```python
from build123d import *

# Parameters (mm, degrees)
SKIZZE1_W   = 5
SKIZZE1_H   = 80
SKIZZE1_W_2 = 50
SKIZZE1_H_2 = 5


with BuildPart() as part:
    # Skizze1 → Rotation1 (revolve)
    with BuildSketch(Plane.XY, mode=Mode.PRIVATE) as rotation1_sk:
        with Locations((-2.5, 40)):
            Rectangle(SKIZZE1_W, SKIZZE1_H)
        with Locations((25, 72.5)):
            Rectangle(SKIZZE1_W_2, SKIZZE1_H_2)
    revolve(rotation1_sk.sketch.rotate(Axis((0, 0, 0), (1, 0, 0)), 90), axis=Axis((0, 0, 0), (1, 0, 0)))


solid = part.part
```
Build history of the part. All positions in model axes, mm. A direction names the side the tool comes from. Give positions to 0.01 mm unless a question says otherwise; leave off trailing zeros. Loops run counter-clockwise (first coordinate to the right, second up) from the corner with the lowest first, then second, coordinate; pieces in that order, holes last.
Item 1: Flat gauge pins, fed straight in: pin 1 (6 mm diameter, centred on y = -34, z = 29.5, fed in from +X); pin 2 (10 mm diameter, centred on x = 31, z = 13.5, fed in from +Y); pin 3 (10 mm diameter, centred on x = 29, y = -0.5, fed in from +Z). Where does each tip first touch, or does it go through?
Answers follow:
pin 1: stops at x = 0
pin 2: stops at y = 74.52
pin 3: stops at z = 75
Item 2: Slice it at A-A, the plane z = 0. List the corners of the cut face in (x, y).
Answers follow:
outline: (-5, -80) - (0, -80) - (0, -75) - (50, -75) - (50, -70) - (0, -70) - (0, 70) - (50, 70) - (50, 75) - (0, 75) - (0, 80) - (-5, 80) - close
Item 3: Drill centre lines: line 1 (Y direction, x = 13, z = 0); line 2 (X direction, y = 44, z = -66.5); line 3 (Y direction, x = 23, z = -19). Where is each one in solid material? Low to high.
Answers follow:
line 1: y = -75 to -70, 70 to 75
line 2: x = -5 to 0
line 3: y = -72.55 to -67.37, 67.37 to 72.55
Item 4: Pull direction Y, two halves, no side cores. Call faces 3 (the face through (-2.465, -3.517, -79.923)), 4 (the face through (25.35, 68.335, -15.175)), 5 (the face through (50, 50, -50)): released by +Y, released by -Y, zero draft, split by the parting line, or undercut.
Answers follow:
face 3: split by the parting line
face 4: undercut
face 5: zero draft
Item 5: Slice it at B-B, the plane x = 28.5. List the corners of the cut face in (y, z), and give its area (3 significant figures).
Answers follow:
outline: circle Ø150 at (0, 0); hole circle Ø140 at (0, 0)
area: 2,280 mm2
Item 6: Which spindle directions (+Z, -Z, +X, -X, +Y, -Y) get a long thin tool onto all of the face, cutting with end or side? Do faces 1 (the face through (-5, -1, 1)), 2 (the face through (25.35, 66.538, 34.608)). Say none if no direction does.
Answers follow:
face 1: +Z, -Z, -X, +Y, -Y
face 2: +X
